from build123d import *

# Parameters (mm, degrees)
F0_W     = 180
F0_H     = 80
F1_DEPTH = 5
F2_R     = 15
F3_R     = 35
F3_R_2   = 25
F3_R_3   = 15
F4_DEPTH = 5


with BuildPart() as f1:
    # F0 (on Top) → F1 (new body, symmetric)
    with BuildSketch(Plane.XY):
        Rectangle(F0_W, F0_H)
    extrude(amount=F1_DEPTH, both=True)

    # F2
    f2_edges = [f1.edges().sort_by_distance(p)[0] for p in [
        (90, 40, 0),
        (-90, 40, 0),
        (90, -40, 0),
        (-90, -40, 0),
    ]]
    fillet(f2_edges, radius=F2_R)

    # F3 (on face) → F4 (cut)
    with BuildSketch(Plane.XY.offset(5)):
        with Locations((-50, 0)):
            Circle(F3_R)
        with Locations((20, 0)):
            Circle(F3_R_2)
        with Locations((70, 0)):
            Circle(F3_R_3)
    extrude(amount=-F4_DEPTH, mode=Mode.SUBTRACT)


solid = f1.part
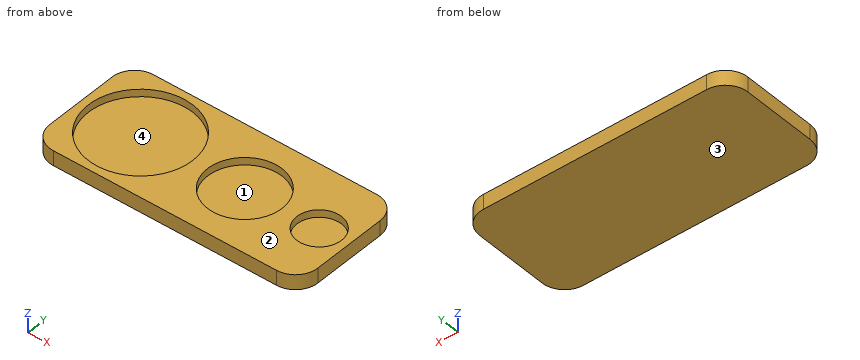
Read the model definition and answer for the solid it produces. Units are mm, in the model's axes. Face numbers are marked on the shaded views. A direction names the side the tool comes from. Coordinates: 2 decimals unless noted, no trailing zeros. Loops run counter-clockwise (first coordinate to the right, second up) from the corner with the lowest first, then second, coordinate; pieces in that order, holes last. Notation, with made-up numbers: (-36, 48) - (21, 48) arc R19 cw to (21, 52) - close; hole circle Ø4 at (84.5, -38). An arc over 180 degrees is marked (long way). Answer in a Markdown table with one row per item.
Q1. Given P1, Ø15, axis at x = 70.5, y = 3.5, coming from the +Z side, flat-ended and moving along its own axis, determine where the tip first touches the part or whether it passes through.
Here are the results:
| item | result |
|---|---|
| P1 | stops at z = 0 |
Q2. Straight lines are drawn through the part: line 1 along Y through (x, z) = (20, 1.45); line 2 along Z through (x, y) = (-78, 14); line 3 along X through (y, z) = (22.5, 1.25). For each, find the intervals that lie inside material, in ascending order. Write a range as [from, to].
Here are the results:
| item | result |
|---|---|
| line 1 | y = [-40, -25], [25, 40] |
| line 2 | z = [-5, 0] |
| line 3 | x = [-90, -76.81], [-23.19, 9.1], [30.9, 90] |
Q3. Find section A-A on x = 70. Write down the section's boundary in (y, z), plus the area to 3 significant figures.
Here are the results:
| item | result |
|---|---|
| outline | (-40, -5) - (40, -5) - (40, 5) - (15, 5) - (15, 0) - (-15, 0) - (-15, 5) - (-40, 5) - close |
| area | 650 mm^2 |
Q4. Find section D-D on x = -50. Write down the section's boundary in (y, z).
Here are the results:
| item | result |
|---|---|
| outline | (-40, -5) - (40, -5) - (40, 5) - (35, 5) - (35, 0) - (-35, 0) - (-35, 5) - (-40, 5) - close |
Q5. Find section B-B on z = 2.5. Write down the section's boundary in (x, y), plus the area to 3 significant figures.
Here are the results:
| item | result |
|---|---|
| outline | (-90, -25) arc R15 ccw to (-75, -40) - (75, -40) arc R15 ccw to (90, -25) - (90, 25) arc R15 ccw to (75, 40) - (-75, 40) arc R15 ccw to (-90, 25) - close; hole circle Ø70 at (-50, 0); hole circle Ø50 at (20, 0); hole circle Ø30 at (70, 0) |
| area | 7,690 mm^2 |
Q6. The mould has two halves that part along X. Classify the marked faces 1 and 2: pulls with the +X half, pulls with the -X half, needs draft (parallel to the pull), parting line crosses it, or undercut.
Here are the results:
| item | result |
|---|---|
| face 1 | undercut |
| face 2 | needs draft |
Q7. Find section C-C on y = 0. Write down the section's boundary in (x, z), plus the area to 3 significant figures.
Here are the results:
| item | result |
|---|---|
| outline | (-90, -5) - (90, -5) - (90, 5) - (85, 5) - (85, 0) - (55, 0) - (55, 5) - (45, 5) - (45, 0) - (-5, 0) - (-5, 5) - (-15, 5) - (-15, 0) - (-85, 0) - (-85, 5) - (-90, 5) - close |
| area | 1,050 mm^2 |
Q8. For the marked faces 3 and 4, determine the directions among +Z, -Z, +X, -X, +Y, -Y from which every point of the face is accessible in a straight line to the end or side of a thin tool.
Here are the results:
| item | result |
|---|---|
| face 3 | -Z, +X, -X, +Y, -Y |
| face 4 | +Z |
